from build123d import *

# Parameters (mm, degrees)
F2_SIZE2      = 10
F2_SIZE       = 10
F3_R          = 6
F4_DEPTH      = 40.001
F4_DEPTH_BACK = 40.001


with BuildPart() as f1:
    # F0 (on Front) → F1 (revolve)
    with BuildSketch(Plane.XZ):
        Polygon((-120, 0), (0, 0), (0, 25), (-90, 25), (-90, 40), (-120, 40), align=None)
    revolve(axis=Axis((-60, 0, 0), (1, 0, 0)))

    # F2
    f2_edges = [f1.edges().sort_by_distance(p)[0] for p in [
        (-120, 0, -40),
        (0, 0, -25),
    ]]
    chamfer(f2_edges, length=F2_SIZE, length2=F2_SIZE2)

    # F3 (on Front) → F4 (cut, two sides)
    with BuildSketch(Plane.XZ) as f4_sk:
        with Locations((-18, 0)):
            Circle(F3_R)
    extrude(amount=-F4_DEPTH, mode=Mode.SUBTRACT)
    extrude(f4_sk.sketch, amount=F4_DEPTH_BACK, mode=Mode.SUBTRACT)


solid = f1.part
Could you check a few things on this model? Use its own coordinates, in mm. A direction names the side the tool comes from. Give positions to 0.01 mm unless a question says otherwise; leave off trailing zeros. Order: outer loops, then holes, each group sorted by start corner. A loop starts at its lowest first (then second) coordinate and runs counter-clockwise, first axis right, second up. Notation, with made-up numbers: M -25,31.25 L 7,31.25 A15 ccw 7,50.25 Z; hole C 20,22 d6. An arc over 180 degrees is marked long. One line per question, with ' | ' between items.
1. I want a section at B-B (x = -18). List the corners of the cut face in (y, z) for me.
Results:
outline: M -24.27,-6 A25 ccw 24.27,-6 Z; M -24.27,6 L 24.27,6 A25 ccw Z
2. I want a section at C-C (x = -106.5). List the corners of the cut face in (y, z) for me, and give its area (3 significant figures).
Results:
outline: C 0,0 d80 | area: 5,030 mm²
3. I want a section at A-A (z = 0). List the corners of the cut face in (x, y) for me, and give its area (3 significant figures).
Results:
outline: M -120,-30 L -110,-40 L -90,-40 L -90,-25 L -24,-25 L -24,25 L -90,25 L -90,40 L -110,40 L -120,30 Z; M -12,-25 L -10,-25 L 0,-15 L 0,15 L -10,25 L -12,25 Z | area: 6,100 mm²
4. I want a section at D-D (x = -62.5). List the corners of the cut face in (y, z) for me, and give its area (3 significant figures).
Results:
outline: C 0,0 d50 | area: 1,960 mm²
5. I'm going to push flat-ended pins straight in: pin 1 (2 mm diameter, centred on x = -41.5, y = -14, fed in from +Z); pin 2 (3 mm diameter, centred on x = -71.5, y = 9, fed in from -Z); pin 3 (11 mm diameter, centred on x = -18, z = 0, fed in from -Y); pin 4 (15.5 mm diameter, centred on x = -18, z = 0, fed in from +Y). Where does each tip first touch, or does it pass through?
Results:
pin 1: z = 21.35 | pin 2: z = -23.85 | pin 3: through | pin 4: y = 25
6. For faces 1 (the face through (-50.6, 22.2, 11.5)), 2 (the face through (-119.51, -9.16, 29.08)), which set-ups out of +Z, -Z, +X, -X, +Y, -Y let a thin tool reach every point of the face, with its end or its side?
Results:
face 1: +X | face 2: -X
7. If I drill on line 1 (X direction, y = -11.25, z = 0); line 2 (Z direction, x = -18, y = 10.75); line 3 (X direction, y = -26, z = 5), over which ranges is the centre line in solid material (lowest first)?
Results:
line 1: -120 to -24, -12 to 0 | line 2: -22.57 to -6, 6 to 22.57 | line 3: -120 to -90
